Verification items for the finished model (mm, model axes). A direction names the side the tool comes from. Round coordinates to 2 decimals unless told otherwise and drop trailing zeros. Write each loop counter-clockwise with the first axis right and the second up, starting at its lowest first coordinate (ties: lowest second). Pieces come first, ordered by that corner, then holes. Notation, with made-up numbers: M 77,74.25 L 119,74.25 A12 ccw 119,95.25 Z; hole C 87.25,-32.5 d7. An arc over 180 degrees is marked long. One line per question, with ' | ' between items.
from build123d import *

# Parameters (mm, degrees)
BOSS_EXTRU_1_DEPTH         = 2.5
ESQUISSE2_R                = 9.5
ENL_V_MAT_EXTRU_1_DEPTH    = 3.5
ESQUISSE3_W                = 4
ESQUISSE3_H                = 7
ENL_V_MAT_EXTRU_2_DEPTH    = 3.5
R_P_TITION_LIN_AIRE1_COUNT = 3
R_P_TITION_LIN_AIRE1_PITCH = 7
ENL_V_MAT_EXTRU_3_DEPTH    = 3.5
ESQUISSE5_W                = 3
ESQUISSE5_H                = 11
ENL_V_MAT_EXTRU_4_DEPTH    = 3.5
R_P_TITION_LIN_AIRE2_COUNT = 2
R_P_TITION_LIN_AIRE2_PITCH = 22
ESQUISSE6_R                = 1.5
ENL_V_MAT_EXTRU_5_DEPTH    = 3.5
ESQUISSE7_W                = 8
ESQUISSE7_H                = 4
ENL_V_MAT_EXTRU_6_DEPTH    = 3.5
SYM_TRIE1_COPY_1_SKETCH_W  = 3
SYM_TRIE1_COPY_1_SKETCH_H  = 11
SYM_TRIE1_COPY_1_DEPTH     = 3.5
SYM_TRIE1_COPY_2_SKETCH_W  = 4
SYM_TRIE1_COPY_2_SKETCH_H  = 7
SYM_TRIE1_COPY_2_DEPTH     = 3.5
SYM_TRIE1_COPY_3_SKETCH_W  = 4
SYM_TRIE1_COPY_3_SKETCH_H  = 7
SYM_TRIE1_COPY_3_DEPTH     = 3.5
ESQUISSE8_R                = 1.5
ENL_V_MAT_EXTRU_7_DEPTH    = 10


with BuildPart() as part:
    # Esquisse1 → Boss.-Extru.1 (new body)
    with BuildSketch(Plane.XY):
        with BuildLine():
            Line((100, 155), (119.994239394, 155))
            ThreePointArc((119.994239394, 155), (121.860222821, 156.2802043), (121.337366241, 158.48189415))
            ThreePointArc((121.337366241, 158.48189415), (50, 186), (-21.337366241, 158.48189415))
            ThreePointArc((-21.337366241, 158.48189415), (-21.860222821, 156.2802043), (-19.994239394, 155))
            Line((-19.994239394, 155), (0, 155))
            Line((0, 155), (0, 0))
            ThreePointArc((0, 0), (50, -14), (100, 0))
            Line((100, 0), (100, 155))
        make_face()
    extrude(amount=BOSS_EXTRU_1_DEPTH)

    # Esquisse2 → Enlèv. mat.-Extru.1 (cut, through all)
    with BuildSketch(Plane(origin=(0, 0, 0), x_dir=(-1, 0, 0), z_dir=(0, 0, -1))):
        with Locations((-50, 155)):
            Circle(ESQUISSE2_R)
    extrude(amount=-ENL_V_MAT_EXTRU_1_DEPTH, mode=Mode.SUBTRACT)

    # Esquisse3 → Enlèv. mat.-Extru.2 (cut, through all)
    with BuildSketch(Plane(origin=(0, 0, 0), x_dir=(-1, 0, 0), z_dir=(0, 0, -1))):
        with Locations((-91, 155)):
            Rectangle(ESQUISSE3_W, ESQUISSE3_H)
    enl_v_mat_extru_2 = extrude(amount=-ENL_V_MAT_EXTRU_2_DEPTH, mode=Mode.SUBTRACT)

    # Répétition linéaire1: Enlèv. mat.-Extru.2 ×3
    with Locations(*[(-i * R_P_TITION_LIN_AIRE1_PITCH, 0, 0) for i in range(1, R_P_TITION_LIN_AIRE1_COUNT)]):
        add(enl_v_mat_extru_2, mode=Mode.SUBTRACT)

    # Esquisse4 → Enlèv. mat.-Extru.3 (cut, through all)
    with BuildSketch(Plane(origin=(0, 0, 0), x_dir=(-1, 0, 0), z_dir=(0, 0, -1))):
        Polygon((-75.5, 122), (-68.5, 122), (-68.5, 115), (-64, 115), (-64, 108), (-68.5, 108), (-68.5, 101), (-75.5, 101), (-75.5, 108), (-80, 108), (-80, 115), (-75.5, 115), align=None)
    enl_v_mat_extru_3 = extrude(amount=-ENL_V_MAT_EXTRU_3_DEPTH, mode=Mode.SUBTRACT)

    # Esquisse5 → Enlèv. mat.-Extru.4 (cut, through all)
    with BuildSketch(Plane(origin=(0, 0, 0), x_dir=(-1, 0, 0), z_dir=(0, 0, -1))):
        with Locations((-78.5, 90.5)):
            Rectangle(ESQUISSE5_W, ESQUISSE5_H)
    enl_v_mat_extru_4 = extrude(amount=-ENL_V_MAT_EXTRU_4_DEPTH, mode=Mode.SUBTRACT)

    # Répétition linéaire2: Enlèv. mat.-Extru.4 ×2
    with Locations(*[(i * R_P_TITION_LIN_AIRE2_PITCH, 0, 0) for i in range(1, R_P_TITION_LIN_AIRE2_COUNT)]):
        add(enl_v_mat_extru_4, mode=Mode.SUBTRACT)

    # Esquisse6 → Enlèv. mat.-Extru.5 (cut, through all)
    with BuildSketch(Plane(origin=(0, 0, 0), x_dir=(-1, 0, 0), z_dir=(0, 0, -1))):
        with Locations((-91, 144.5)):
            Circle(ESQUISSE6_R)
        with Locations((-91, 124.5)):
            Circle(ESQUISSE6_R)
        with Locations((-65, 17.5)):
            Circle(ESQUISSE6_R)
        with Locations((-69, 26.5)):
            Circle(ESQUISSE6_R)
        with Locations((-91.030029605, 0.602552335)):
            Circle(ESQUISSE6_R)
        with Locations((-77.401365798, -2.600496654)):
            Circle(ESQUISSE6_R)
        with Locations((-69, 4.5)):
            Circle(ESQUISSE6_R)
        with Locations((-65, -6.5)):
            Circle(ESQUISSE6_R)
        with Locations((-69, 62.5)):
            Circle(ESQUISSE6_R)
        with BuildLine():
            Line((-82, 54.5), (-82, 44.5))
            ThreePointArc((-82, 44.5), (-83.5, 43), (-85, 44.5))
            Line((-85, 44.5), (-85, 54.5))
            ThreePointArc((-85, 54.5), (-83.5, 56), (-82, 54.5))
        make_face()
        with BuildLine():
            Line((-74, 51), (-64, 51))
            ThreePointArc((-64, 51), (-62.5, 49.5), (-64, 48))
            Line((-64, 48), (-74, 48))
            ThreePointArc((-74, 48), (-75.5, 49.5), (-74, 51))
        make_face()
        with BuildLine():
            Line((-82, 136.5), (-82, 126.5))
            ThreePointArc((-82, 126.5), (-83.5, 125), (-85, 126.5))
            Line((-85, 126.5), (-85, 136.5))
            ThreePointArc((-85, 136.5), (-83.5, 138), (-82, 136.5))
        make_face()
        with BuildLine():
            Line((-113.087366241, 159.299038106), (-76.714299282, 180.299038106))
            ThreePointArc((-76.714299282, 180.299038106), (-74.665261177, 179.75), (-75.214299282, 177.700961894))
            Line((-75.214299282, 177.700961894), (-111.587366241, 156.700961894))
            ThreePointArc((-111.587366241, 156.700961894), (-113.636404347, 157.25), (-113.087366241, 159.299038106))
        make_face()
    enl_v_mat_extru_5 = extrude(amount=-ENL_V_MAT_EXTRU_5_DEPTH, mode=Mode.SUBTRACT)

    # Esquisse7 → Enlèv. mat.-Extru.6 (cut, through all)
    with BuildSketch(Plane(origin=(0, 0, 0), x_dir=(-1, 0, 0), z_dir=(0, 0, -1))):
        with Locations((-89, 37)):
            Rectangle(ESQUISSE7_W, ESQUISSE7_H)
        with Locations((-89, 30)):
            Rectangle(ESQUISSE7_W, ESQUISSE7_H)
        with Locations((-89, 23)):
            Rectangle(ESQUISSE7_W, ESQUISSE7_H)
    enl_v_mat_extru_6 = extrude(amount=-ENL_V_MAT_EXTRU_6_DEPTH, mode=Mode.SUBTRACT)

    # Symétrie1: Enlèv. mat.-Extru.2, Enlèv. mat.-Extru.3, Enlèv. mat.-Extru.4, Enlèv. mat.-Extru.5, Enlèv. mat.-Extru.6 across plane
    add(enl_v_mat_extru_2.mirror(Plane(origin=(50, 0, 0), x_dir=(0, 0, 1), z_dir=(1, 0, 0))), mode=Mode.SUBTRACT)
    add(enl_v_mat_extru_3.mirror(Plane(origin=(50, 0, 0), x_dir=(0, 0, 1), z_dir=(1, 0, 0))), mode=Mode.SUBTRACT)
    add(enl_v_mat_extru_4.mirror(Plane(origin=(50, 0, 0), x_dir=(0, 0, 1), z_dir=(1, 0, 0))), mode=Mode.SUBTRACT)
    add(enl_v_mat_extru_5.mirror(Plane(origin=(50, 0, 0), x_dir=(0, 0, 1), z_dir=(1, 0, 0))), mode=Mode.SUBTRACT)
    add(enl_v_mat_extru_6.mirror(Plane(origin=(50, 0, 0), x_dir=(0, 0, 1), z_dir=(1, 0, 0))), mode=Mode.SUBTRACT)

    # Symétrie1 copy 1 sketch → Symétrie1 copy 1 (cut, through all)
    with BuildSketch(Plane(origin=(78, 0, 0), x_dir=(1, 0, 0), z_dir=(0, 0, -1))):
        with Locations((-78.5, -90.5)):
            Rectangle(SYM_TRIE1_COPY_1_SKETCH_W, SYM_TRIE1_COPY_1_SKETCH_H)
    extrude(amount=-SYM_TRIE1_COPY_1_DEPTH, mode=Mode.SUBTRACT)

    # Symétrie1 copy 2 sketch → Symétrie1 copy 2 (cut, through all)
    with BuildSketch(Plane(origin=(107, 0, 0), x_dir=(1, 0, 0), z_dir=(0, 0, -1))):
        with Locations((-91, -155)):
            Rectangle(SYM_TRIE1_COPY_2_SKETCH_W, SYM_TRIE1_COPY_2_SKETCH_H)
    extrude(amount=-SYM_TRIE1_COPY_2_DEPTH, mode=Mode.SUBTRACT)

    # Symétrie1 copy 3 sketch → Symétrie1 copy 3 (cut, through all)
    with BuildSketch(Plane(origin=(114, 0, 0), x_dir=(1, 0, 0), z_dir=(0, 0, -1))):
        with Locations((-91, -155)):
            Rectangle(SYM_TRIE1_COPY_3_SKETCH_W, SYM_TRIE1_COPY_3_SKETCH_H)
    extrude(amount=-SYM_TRIE1_COPY_3_DEPTH, mode=Mode.SUBTRACT)

    # Esquisse8 → Enlèv. mat.-Extru.7 (cut)
    with BuildSketch(Plane(origin=(0, 0, 0), x_dir=(-1, 0, 0), z_dir=(0, 0, -1))):
        with Locations((-50, 111.5)):
            Circle(ESQUISSE8_R)
        with Locations((-50, 125)):
            Circle(ESQUISSE8_R)
        with Locations((-50, 98)):
            Circle(ESQUISSE8_R)
        with Locations((-50, 71)):
            Circle(ESQUISSE8_R)
        with Locations((-50, -8)):
            Circle(ESQUISSE8_R)
        with Locations((-50, 11)):
            Circle(ESQUISSE8_R)
        with BuildLine():
            Line((-67.5, 180.480620573), (-32.5, 180.480620573))
            ThreePointArc((-32.5, 180.480620573), (-31, 178.980620573), (-32.5, 177.480620573))
            Line((-32.5, 177.480620573), (-67.5, 177.480620573))
            ThreePointArc((-67.5, 177.480620573), (-69, 178.980620573), (-67.5, 180.480620573))
        make_face()
    extrude(amount=-ENL_V_MAT_EXTRU_7_DEPTH, mode=Mode.SUBTRACT)


solid = part.part
1. Mould release check, pull along X, two halves, no side actions. Record for faces 1 (the face through (49, 87, 2.5)), 2 (the face through (49.264, -13.997, 1.232)), 3 (the face through (6.854, 167.348, 1.232)): pulls with the +X half, pulls with the -X half, needs draft (parallel to the pull), parting line crosses it, or undercut.
Results:
face 1: needs draft | face 2: parting line crosses it | face 3: undercut
2. Tool access check on faces 4 (the face through (4.84, 169.65, 1.23)), 5 (the face through (51.095, 185.994, 1.232)). Record the directions out of +Z, -Z, +X, -X, +Y, -Y that give a thin tool (end or side, any length) a straight path to the whole face; none if there is none.
Results:
face 4: +Z, -Z | face 5: +Z, -Z, +Y
3. Section check B-B, the plane z = 1.4. Count the separate pieces of the cut face and the enclosed holes in it, then the cut area to 3 significant figures.
Results:
separate pieces: 1 | enclosed holes: 50 | area: 17,700 mm2
4. Go/stop test with flat-tipped pins: P1, Ø0.8, axis at x = 23.5, z = 1.5, coming from the -Y side; P2, Ø0.8, axis at x = 8, z = 1.5, coming from the +Y side; P3, Ø0.8, axis at y = 90, z = 1, coming from the +X side. Record where each tip stops, or that it passes through.
Results:
P1: stops at y = -10.4 | P2: stops at y = 177.52 | P3: stops at x = 99
5. Thickness scan on line 1 (X direction, y = 92, z = 2.15); line 2 (X direction, y = 49.5, z = 1.4); line 3 (X direction, y = 63, z = 0.6). Record the ranges inside material, lowest first.
Results:
line 1: x = 1 to 20, 23 to 77, 80 to 99 | line 2: x = 0 to 15, 18 to 24.5, 37.5 to 62.5, 75.5 to 82, 85 to 100 | line 3: x = 0 to 29.59, 32.41 to 67.59, 70.41 to 100
6. Section check A-A, the plane x = 45.5. Record the cut outline in (y, z), then the cut area to 3 significant figures.
Results:
outline: M -13.89,0 L 146.63,0 L 146.63,2.5 L -13.89,2.5 Z; M 163.37,0 L 177.48,0 L 177.48,2.5 L 163.37,2.5 Z; M 180.48,0 L 185.9,0 L 185.9,2.5 L 180.48,2.5 Z | area: 450 mm2
